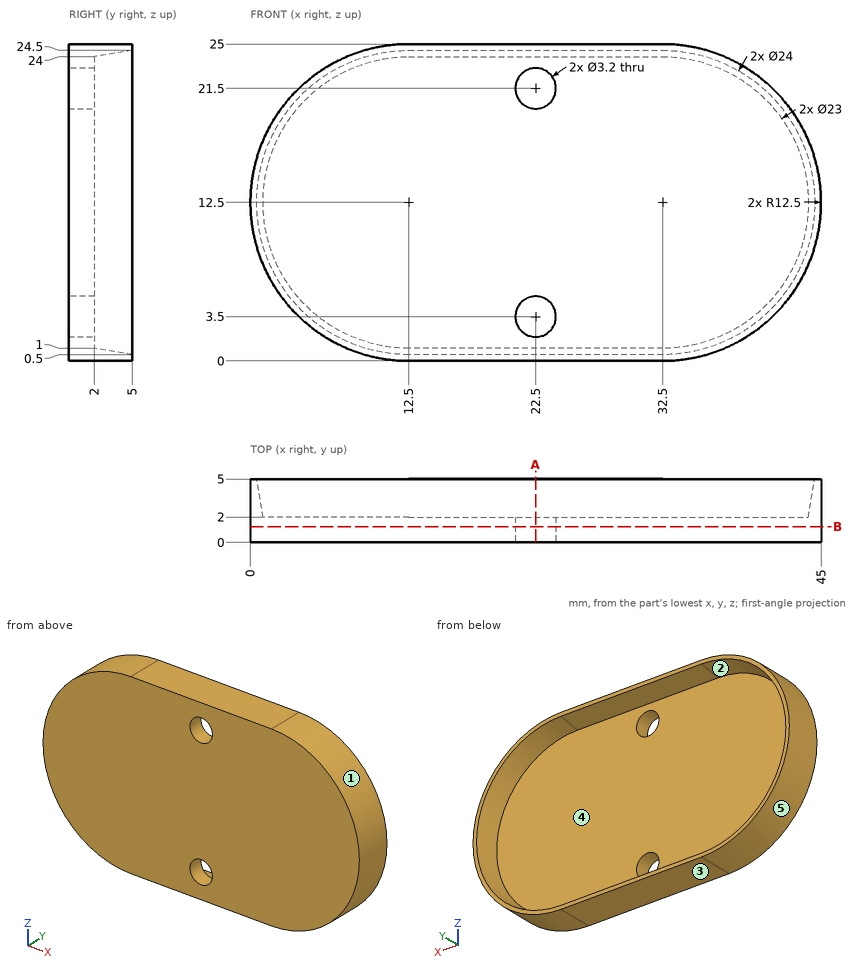
Geometry check sheet. Reference: drawing and pictorial views, mm from the part's lowest x, y, z. A direction names the side the tool comes from. Coordinates: 2 decimals unless noted, no trailing zeros. Loops run counter-clockwise (first coordinate to the right, second up) from the corner with the lowest first, then second, coordinate; pieces in that order, holes last.
1) Access from +Z, -Z, +X, -X, +Y, -Y to the whole of each face (thin tool, end or side, straight path). Record for the marked faces 1 and 2.
2) Release check for a two-part mould opening along Z. For the marked faces 3, 4 and 5 record: released by +Z, released by -Z, zero draft, split by the parting line, or undercut.
3) Gauge pin test, flat ends, axial feed: pin 1 (1 mm diameter, centred on y = 2.5, z = 10.5, fed in from +X); pin 2 (1 mm diameter, centred on x = 19, z = 7, fed in from +Y); pin 3 (3 mm diameter, centred on y = 3, z = 15.5, fed in from -X); pin 4 (2.5 mm diameter, centred on x = 22.5, z = 3.5, fed in from +Y). Record the tip position at first contact, or that the pin passes through.
4) Material ranges on probe 1 along Y at (x, z) = (10, 5.75); probe 2 along Z at (x, y) = (23, 1.35); probe 3 along X at (y, z) = (4.7, 1.5), recorded low to high.
5) Sectioned sample at A-A (x = 22.5). Record the boundary of the cut face in (y, z), and give its area (3 significant figures).
6) Sectioned sample at B-B (y = 1.25). Record the boundary of the cut face in (x, z), and give its area (3 significant figures).
Check sheet entries:
1. face 1: +X, +Y, -Y
1. face 2: +Y
2. face 3: released by -Z
2. face 4: undercut
2. face 5: split by the parting line
3. pin 1: stops at x = 44.91
3. pin 2: stops at y = 2
3. pin 3: stops at x = 0.09
3. pin 4: passes through
4. probe 1: y = 0 to 2
4. probe 2: z = 0 to 1.98, 5.02 to 19.98, 23.02 to 25
4. probe 3: x = 6.56 to 7.83, 37.17 to 38.44
5. outline: (0, 0) - (5, 0) - (5, 0.5) - (2, 1) - (2, 1.9) - (0, 1.9) - close; (0, 5.1) - (2, 5.1) - (2, 19.9) - (0, 19.9) - close; (0, 23.1) - (2, 23.1) - (2, 24) - (5, 24.5) - (5, 25) - (0, 25) - close
5. area: 41.7 mm2
6. outline: (12.5, 0) - (32.5, 0) arc R12.5 ccw to (32.5, 25) - (12.5, 25) arc R12.5 ccw to start; hole circle Ø3.2 at (22.5, 3.5); hole circle Ø3.2 at (22.5, 21.5)
6. area: 975 mm2
